For this review, take the finished solid that the model builds, in its own axes (mm). Round coordinates to 2 decimals unless told otherwise and drop trailing zeros. Loops run counter-clockwise (first coordinate to the right, second up) from the corner with the lowest first, then second, coordinate; pieces in that order, holes last.
1) Insertion check: pin 1 (2.5 mm diameter, centred on x = -28.38, y = 10.48, fed in from +Z). The pin has a flat end and moves straight along its axis. Give the tip position at first contact, or say it passes through.
2) Mouldability with a two-part tool opening along X and no side actions: class faces 1 (the cylindrical face through (-27.024, -11.042, 3.131)), 2 (the flat face through (-38.1, 0, 3)), 3 (the flat face through (12, 17.462, 3)) as pulls with the +X half, pulls with the -X half, needs draft (parallel to the pull), parting line crosses it, or undercut.
3) Take a section at C-C (y = 4.5). State the section outline as (x, z) points.
4) Wall thickness on L1, parallel to Y at x = 28.5, z = 0.75; L2, parallel to X at y = 10.5, z = 4.75; L3, parallel to X at y = 10, z = 5: over which ranges is each line inside the solid? List them lowest first.
5) Take a section at B-B (z = 3). State the section outline as (x, y) points.
6) Take a section at A-A (y = 0). State the section outline as (x, z) points, then the cut area to 3 significant figures.
```python
from build123d import *

# Parameters (mm, degrees)
SKETCH1_W               = 101.6
SKETCH1_H               = 34.925
BOSS_EXTRUDE1_DEPTH     = 6.35
ADVANCEDHOLE1_OUTLINE_R = 1.4732
ADVANCEDHOLE1_DEPTH     = 6.35
CUT_EXTRUDE1_REACH      = 68.163
SKETCH5_R               = 6.35


# Read off the part's stored shape, not the designer's step: AdvancedHole1
with BuildPart() as part:
    # Sketch1 → Boss-Extrude1 (new body)
    with BuildSketch(Plane.XY):
        with Locations((12.7, 0)):
            Rectangle(SKETCH1_W, SKETCH1_H)
    extrude(amount=BOSS_EXTRUDE1_DEPTH)

    # AdvancedHole1 outline → AdvancedHole1 (cut)
    with BuildSketch(Plane.XY):
        with Locations((28.3845, 10.4775)):
            Circle(ADVANCEDHOLE1_OUTLINE_R)
        with Locations((28.3845, -10.4775)):
            Circle(ADVANCEDHOLE1_OUTLINE_R)
        with Locations((-28.3845, -10.4775)):
            Circle(ADVANCEDHOLE1_OUTLINE_R)
        with Locations((-28.3845, 10.4775)):
            Circle(ADVANCEDHOLE1_OUTLINE_R)
    extrude(amount=ADVANCEDHOLE1_DEPTH, mode=Mode.SUBTRACT)

    # Sketch5 → Cut-Extrude1 (cut, up to next)
    with BuildSketch(Plane.XY.offset(6.35), mode=Mode.PRIVATE) as cut_extrude1_sk1:
        with Locations((15.6845, 0)):
            Circle(SKETCH5_R)
    cut_extrude1_tool1 = extrude(cut_extrude1_sk1.sketch, amount=-CUT_EXTRUDE1_REACH, mode=Mode.PRIVATE) & part.part
    add(cut_extrude1_tool1.solids().sort_by_distance((15.6845, 0, 6.35))[0], mode=Mode.SUBTRACT)


solid = part.part
```
Response:
1. pin 1: passes through
2. face 1: undercut
2. face 2: pulls with the -X half
2. face 3: needs draft
3. outline: (-38.1, 0) - (11.2, 0) - (11.2, 6.35) - (-38.1, 6.35) - close; (20.16, 0) - (63.5, 0) - (63.5, 6.35) - (20.16, 6.35) - close
4. L1: y = -17.46 to -11.95, -9.01 to 9.01, 11.95 to 17.46
4. L2: x = -38.1 to -29.86, -26.91 to 26.91, 29.86 to 63.5
4. L3: x = -38.1 to -29.78, -26.99 to 26.99, 29.78 to 63.5
5. outline: (-38.1, -17.46) - (63.5, -17.46) - (63.5, 17.46) - (-38.1, 17.46) - close; hole circle Ø2.95 at (-28.38, -10.48); hole circle Ø2.95 at (-28.38, 10.48); hole circle Ø12.7 at (15.68, 0); hole circle Ø2.95 at (28.38, -10.48); hole circle Ø2.95 at (28.38, 10.48)
6. outline: (-38.1, 0) - (9.33, 0) - (9.33, 6.35) - (-38.1, 6.35) - close; (22.03, 0) - (63.5, 0) - (63.5, 6.35) - (22.03, 6.35) - close
6. area: 565 mm2
